Here's the drawing with two shaded views (mm, measured from the low corner). I have some questions. A direction names the side the tool comes from. Give positions to 0.01 mm unless a question says otherwise; leave off trailing zeros. Loops run counter-clockwise (first coordinate to the right, second up) from the corner with the lowest first, then second, coordinate; pieces in that order, holes last.
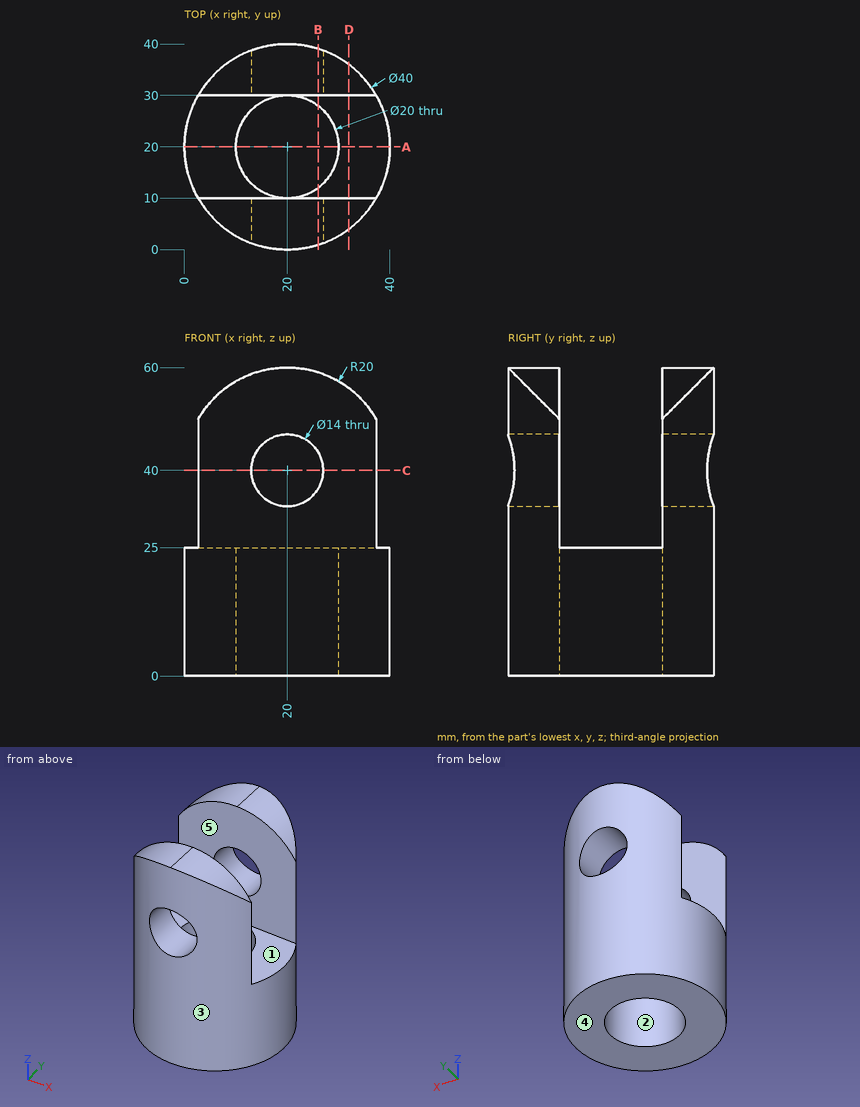
(1) Suppose I cut it at D-D on x = 32. List the corners of the cut face in (y, z) for me.
Returned:
outline: (4, 0) - (36, 0) - (36, 56) - (30, 56) - (30, 25) - (10, 25) - (10, 56) - (4, 56) - close
(2) Suppose I cut it at C-C on z = 40. List the corners of the cut face in (x, y) for me (1 decimal), plus the area to 3 significant figures.
Returned:
outline: (2.7, 10) arc R20 ccw to (13, 1.3) - (13, 10) - close; (2.7, 30) - (13, 30) - (13, 38.7) arc R20 ccw to start; (27, 1.3) arc R20 ccw to (37.3, 10) - (27, 10) - close; (27, 30) - (37.3, 30) arc R20 ccw to (27, 38.7) - close
area: 223 mm2
(3) Will these pins go through, and if not, where does the flat tip stop? P1, Ø1.5, axis at x = 21.5, z = 23, coming from the -Y side; P2, Ø3, axis at x = 33, z = 9.5, coming from the -Y side; P3, Ø10, axis at x = 20, y = 16, coming from the +Z side; P4, Ø3, axis at y = 29, z = 24.5, coming from the +X side.
Returned:
P1: stops at y = 0.01
P2: stops at y = 3.64
P3: passes through
P4: stops at x = 38.54
(4) Suppose I cut it at B-B on x = 26. List the corners of the cut face in (y, z) for me.
Returned:
outline: (0.92, 0) - (12, 0) - (12, 25) - (10, 25) - (10, 36.39) - (0.92, 36.39) - close; (0.92, 43.61) - (10, 43.61) - (10, 59.08) - (0.92, 59.08) - close; (28, 0) - (39.08, 0) - (39.08, 36.39) - (30, 36.39) - (30, 25) - (28, 25) - close; (30, 43.61) - (39.08, 43.61) - (39.08, 59.08) - (30, 59.08) - close
(5) Please list where these lines run through material, in increasing order: probe 1 along Y at (x, z) = (20, 10); probe 2 along Z at (x, y) = (9.5, 21.5); probe 3 along X at (y, z) = (34, 40).
Returned:
probe 1: y = 0 to 10, 30 to 40
probe 2: z = 0 to 25
probe 3: x = 5.72 to 13, 27 to 34.28
(6) Thinking about a two-plate mould opening in X: for the marked faces 1, 2 and 3, which applies, pulls with the +X half, pulls with the -X half, needs draft (parallel to the pull), parting line crosses it, or undercut?
Returned:
face 1: needs draft
face 2: undercut
face 3: parting line crosses it
(7) Which directions (+Z, -Z, +X, -X, +Y, -Y) give clear straight access to the entire face, cutting with the end or side of a thin tool? Please do the marked faces 4 and 5.
Returned:
face 4: -Z, +X, -X, +Y, -Y
face 5: +Z, +X, -X
(8) Suppose I cut it at A-A on y = 20. List the corners of the cut face in (x, z) for me.
Returned:
outline: (0, 0) - (10, 0) - (10, 25) - (0, 25) - close; (30, 0) - (40, 0) - (40, 25) - (30, 25) - close
